```python
from build123d import *

# Parameters (mm, degrees)
F0_R     = 76.88013
F1_DEPTH = 65.278
F2_R     = 25.084702
F3_DEPTH = 25.4
F4_R     = 5.08
F5_R     = 20.32


with BuildPart() as f1:
    # F0 (on Top) → F1 (new body)
    with BuildSketch(Plane.XY):
        Circle(F0_R)
    extrude(amount=F1_DEPTH)

    # F2 (on face) → F3 (join)
    with BuildSketch(Plane.XY.offset(65.278)):
        Circle(F2_R)
    extrude(amount=F3_DEPTH)

    # F4
    f4_edges = [f1.edges().sort_by_distance(p)[0] for p in [
        (-76.88013, 0, 0),
    ]]
    fillet(f4_edges, radius=F4_R)

    # F5
    f5_edges = [f1.edges().sort_by_distance(p)[0] for p in [
        (-76.88013, 0, 65.278),
    ]]
    fillet(f5_edges, radius=F5_R)


solid = f1.part
```
Geometry: final body of the model. Coordinates: model frame, mm. A direction names the side the tool comes from. Round coordinates to 2 decimals unless told otherwise and drop trailing zeros. Loops run counter-clockwise (first coordinate to the right, second up) from the corner with the lowest first, then second, coordinate; pieces in that order, holes last. Notation, with made-up numbers: (45, -4) -> (103, -4) arc R18 cw to (103, 8) -> close; hole circle Ø11 at (14, 44.25). An arc over 180 degrees is marked (long way). Write each question's results on one line, items separated by ' | '.
Item 1: Cut plane C-C on z = 35.5. Return the cut outline in (x, y), and give its area (3 significant figures).
Answers below:
outline: circle Ø153.76 at (0, 0) | area: 18,600 mm²
Item 2: Cut plane D-D on z = 76. Return the cut outline in (x, y).
Answers below:
outline: circle Ø50.17 at (0, 0)
Item 3: Cut plane A-A on x = 0. Return the cut outline in (y, z).
Answers below:
outline: (-76.88, 5.08) arc R5.08 ccw to (-71.8, 0) -> (71.8, 0) arc R5.08 ccw to (76.88, 5.08) -> (76.88, 44.96) arc R20.32 ccw to (56.56, 65.28) -> (25.08, 65.28) -> (25.08, 90.68) -> (-25.08, 90.68) -> (-25.08, 65.28) -> (-56.56, 65.28) arc R20.32 ccw to (-76.88, 44.96) -> close
Item 4: Line query: probe 1 along Z at (x, y) = (10, 54); probe 2 along X at (y, z) = (2, 14); probe 3 along X at (y, z) = (37, 30). Output: solid intervals per line, ascending. Write a range as [from, to].
Answers below:
probe 1: z = [0, 65.28] | probe 2: x = [-76.85, 76.85] | probe 3: x = [-67.39, 67.39]
Item 5: Set-up query: faces 1 (the face through (-1, 1, 0)), 2 (the face through (24, -12, 65.278)). Return all of +Z, -Z, +X, -X, +Y, -Y with unobstructed straight access to the full face (end or side cutting, diameter ignored); none if empty.
Answers below:
face 1: -Z, +X, -X, +Y, -Y | face 2: +Z
Item 6: Pin query (flat end, axial travel): pin 1 Ø1.5 at (x, z) = (-10, 71) entering from -Y; pin 2 Ø2 at (x, z) = (0.5, 27.5) entering from -Y; pin 3 Ø2 at (y, z) = (-23, 60) entering from -X. Return the tip coordinate at first contact, or that it passes through.
Answers below:
pin 1: stops at y = -23.32 | pin 2: stops at y = -76.88 | pin 3: stops at x = -67.49
